Geometry check sheet. Reference: the model listing, model coordinates, mm. Face numbers are marked on the shaded views. A direction names the side the tool comes from. Round coordinates to 2 decimals unless told otherwise and drop trailing zeros. Write each loop counter-clockwise with the first axis right and the second up, starting at its lowest first coordinate (ties: lowest second). Pieces come first, ordered by that corner, then holes.
Item 1: Cross-section at C-C (x = -14.5). Enter the section's corners in (y, z), then the cut area to 3 significant figures.
Item 2: Depth check by flat-ended pin: P1, Ø5, axis at x = 133.5, y = 11, coming from the +Z side; P2, Ø5, axis at y = 15.5, z = 3, coming from the -X side; P3, Ø8, axis at x = 140, y = -3.5, coming from the +Z side. Enter the tip coordinate at first touch or a pass-through.
Item 3: Cross-section at A-A (y = 0). Enter the section's corners in (x, z), then the cut area to 3 significant figures.
Item 4: Cross-section at D-D (x = 74). Enter the section's corners in (y, z), then the cut area to 3 significant figures.
Item 5: Scan lines: probe 1 along X at (y, z) = (13, -9); probe 2 along Z at (x, y) = (-55.5, 7); probe 3 along Z at (x, y) = (216, 3.5). Record each from-to range of solid material in increasing order.
Item 6: Access from +Z, -Z, +X, -X, +Y, -Y to the whole of each face (thin tool, end or side, straight path). Record for the marked faces 1, 2 and 3.
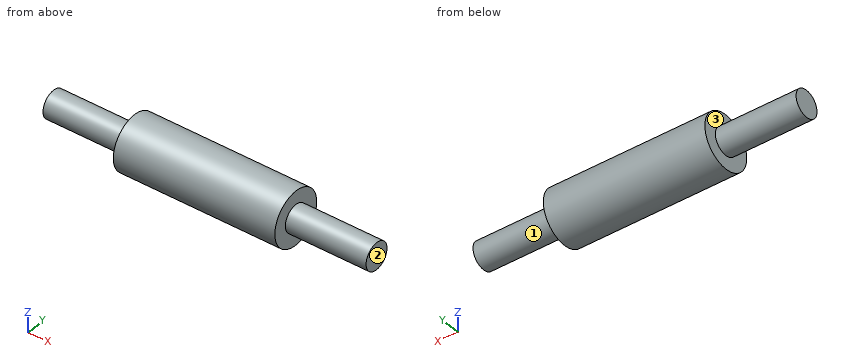
from build123d import *

# Parameters (mm, degrees)
F0_R     = 25.4
F1_DEPTH = 152.4
F2_R     = 12.7
F3_DEPTH = 76.2
F4_R     = 12.7
F5_DEPTH = 76.2


with BuildPart() as f1:
    # F0 (on Right) → F1 (new body)
    with BuildSketch(Plane.YZ):
        Circle(F0_R)
    extrude(amount=F1_DEPTH)

    # F2 (on face) → F3 (join)
    with BuildSketch(Plane(origin=(0, 0, 0), x_dir=(0, -1, 0), z_dir=(-1, 0, 0))):
        Circle(F2_R)
    extrude(amount=F3_DEPTH)

    # F4 (on face) → F5 (join)
    with BuildSketch(Plane.YZ.offset(152.4)):
        Circle(F4_R)
    extrude(amount=F5_DEPTH)


solid = f1.part
Resolved:
1. outline: circle Ø25.4 at (0, 0)
1. area: 507 mm2
2. P1: stops at z = 23.94
2. P2: stops at x = 0
2. P3: stops at z = 25.4
3. outline: (-76.2, -12.7) - (0, -12.7) - (0, -25.4) - (152.4, -25.4) - (152.4, -12.7) - (228.6, -12.7) - (228.6, 12.7) - (152.4, 12.7) - (152.4, 25.4) - (0, 25.4) - (0, 12.7) - (-76.2, 12.7) - close
3. area: 11,600 mm2
4. outline: circle Ø50.8 at (0, 0)
4. area: 2,030 mm2
5. probe 1: x = 0 to 152.4
5. probe 2: z = -10.6 to 10.6
5. probe 3: z = -12.21 to 12.21
6. face 1: +X
6. face 2: +Z, -Z, +X, +Y, -Y
6. face 3: -X
